Read the model definition and answer for the solid it produces. Units are mm, in the model's axes. Face numbers are marked on the shaded views. A direction names the side the tool comes from. Give positions to 0.01 mm unless a question says otherwise; leave off trailing zeros. Order: outer loops, then holes, each group sorted by start corner. A loop starts at its lowest first (then second) coordinate and runs counter-clockwise, first axis right, second up. Notation, with made-up numbers: (54.25, -6.5) - (94.25, -6.5) arc R8 ccw to (94.25, 4.5) - close; hole circle Ø10 at (77, 85). An arc over 180 degrees is marked (long way). Write item = value, one per line.
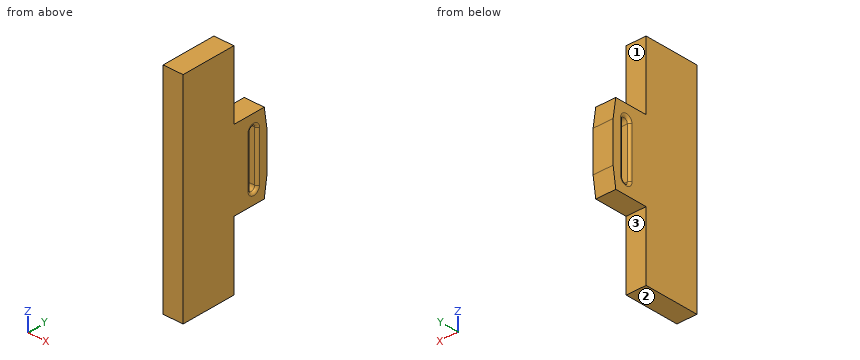
```python
from build123d import *
from OCP.BRepAlgoAPI import BRepAlgoAPI_Cut
from OCP.TopTools import TopTools_ListOfShape

# Parameters (mm, degrees)
SKETCH_1_W          = 86
SKETCH_1_H          = 44.920858062
EXTRUDE_1_DEPTH     = 8
CUT_EXTRUDE_2_DEPTH = 92.635829898
CUT_EXTRUDE_3_DEPTH = 90.129115951
FILLET_1_R          = 1


with BuildPart() as part:
    # Эскиз1 → Вытянуть1 (new body)
    with BuildSketch(Plane(origin=(0, 0, 0), x_dir=(0, 0, -1), z_dir=(1, 0, 0))):
        with Locations((43, -8.152073661)):
            Rectangle(SKETCH_1_W, SKETCH_1_H)
    extrude(amount=EXTRUDE_1_DEPTH)


with BuildPart() as cut_extrude_2_tool:
    # Эскиз3 → Вырез-Вытянуть2 (new, through all)
    with BuildSketch(Plane.ZY):
        Polygon((0, -30.612502692), (-2.2e-07, -21.999984323), (-86, -21.999984323), (-86, -30.612502692), align=None)
        Polygon((0, 14.387497308), (-3.68e-07, 0), (-27.157261974, 0), (-27.157261974, 13.148042163), (-35.5, 14.387497308), align=None)
        Polygon((-58.842738026, 0), (-58.842738026, 13.148042163), (-50.5, 14.387497308), (-86, 14.387497308), (-85.999999632, 0), align=None)
    extrude(amount=-CUT_EXTRUDE_2_DEPTH)


with BuildPart() as part_1:
    add(part.part)

    # Вырез-Вытянуть2: cut by cut_extrude_2_tool, with a tolerance
    cut_extrude_2_stock = TopTools_ListOfShape()
    cut_extrude_2_stock.Append(part_1.part.wrapped)
    cut_extrude_2_tools = TopTools_ListOfShape()
    cut_extrude_2_tools.Append(cut_extrude_2_tool.part.wrapped)
    cut_extrude_2_cut = BRepAlgoAPI_Cut()
    cut_extrude_2_cut.SetArguments(cut_extrude_2_stock)
    cut_extrude_2_cut.SetTools(cut_extrude_2_tools)
    cut_extrude_2_cut.SetFuzzyValue(0.00001)
    cut_extrude_2_cut.Build()
    add(Compound.cast(cut_extrude_2_cut.Shape()).solids(), mode=Mode.REPLACE)

    # Эскиз4 → Вырез-Вытянуть3 (cut, through all)
    with BuildSketch(Plane.ZY):
        with BuildLine():
            Line((-53.089945506, 10.085003592), (-33.089945506, 10.085003592))
            ThreePointArc((-33.089945506, 10.085003592), (-31.589945506, 8.585003592), (-33.089945506, 7.085003592))
            Line((-33.089945506, 7.085003592), (-53.089945506, 7.085003592))
            ThreePointArc((-53.089945506, 7.085003592), (-54.589945506, 8.585003592), (-53.089945506, 10.085003592))
        make_face()
    extrude(amount=-CUT_EXTRUDE_3_DEPTH, mode=Mode.SUBTRACT)

    # Скругление1
    fillet_1_edges = [part_1.edges().sort_by_distance(p)[0] for p in [
        (8, 8.585003592, -54.589945506),
        (8, 10.085003592, -43.089945506),
        (8, 8.585003592, -31.589945506),
        (8, 7.085003592, -43.089945506),
        (0, 8.585003592, -54.589945506),
        (0, 7.085003592, -43.089945506),
        (0, 8.585003592, -31.589945506),
        (0, 10.085003592, -43.089945506),
    ]]
    fillet(fillet_1_edges, radius=FILLET_1_R)


solid = part_1.part
```
1. Flat-ended cylindrical pins translate along their axes: pin 1 (4 mm diameter, centred on x = 3, z = -71, fed in from +Y); pin 2 (2 mm diameter, centred on x = 5, y = 2, fed in from +Z). Find the tip coordinate at first contact, or state that the pin passes through.
Recorded:
pin_1 = 0
pin_2 = -27.16
2. Straight lines are drawn through the part: L1, parallel to Y at x = 2.25, z = -44 (3 decimals); L2, parallel to Y at x = 1.75, z = -26; L3, parallel to Z at x = 1.25, y = 11.5. For each, find the intervals that lie inside material, in ascending order. Write a range as [from, to].
Recorded:
L1 = [-22, 7.085], [10.085, 14.308]
L2 = [-22, 0]
L3 = [-58.84, -27.16]
3. For the marked faces 1, 2 and 3, determine the directions among +Z, -Z, +X, -X, +Y, -Y from which every point of the face is accessible in a straight line to the end or side of a thin tool.
Recorded:
face_1 = +Z, +X, -X, +Y
face_2 = -Z, +X, -X, +Y, -Y
face_3 = -Z, +X, -X, +Y
4. Section A-A (x = 3) is taken. Determine the outline of the cut face in (y, z) (3 decimals), and give its area (3 significant figures).
Recorded:
outline = (-22, -86) - (0, -86) - (0, -58.843) - (13.148, -58.843) - (14.308, -51.033) - (14.308, -34.967) - (13.148, -27.157) - (0, -27.157) - (0, 0) - (-22, 0) - close; hole (7.085, -53.09) arc R1.5 ccw to (10.085, -53.09) - (10.085, -33.09) arc R1.5 ccw to (7.085, -33.09) - close
area = 2,270 mm^2
5. Section B-B (z = -65) is taken. Determine the outline of the cut face in (x, y), and give its area (3 significant figures).
Recorded:
outline = (0, -22) - (8, -22) - (8, 0) - (0, 0) - close
area = 176 mm^2
6. Section C-C (y = 3) is taken. Determine the outline of the cut face in (x, z).
Recorded:
outline = (0, -58.84) - (8, -58.84) - (8, -27.16) - (0, -27.16) - close
